Design review of the part built by this model. Coordinates are the model's own, in mm. A direction names the side the tool comes from. Coordinates: 2 decimals unless noted, no trailing zeros. Write each loop counter-clockwise with the first axis right and the second up, starting at its lowest first coordinate (ties: lowest second). Pieces come first, ordered by that corner, then holes.
Q1. Take a section at A-A (x = 29.5). Give the boundary of the cut face in (y, z), and give its area (3 significant figures).
Q2. Mouldability with a two-part tool opening along Z and no side actions: class faces 1 (the flat face through (-0.2, 17.4, 0)), 2 (the cylindrical face through (27.75, 0.99, 10.08)), 3 (the flat face through (-34, 1, 10)) as pulls with the +Z half, pulls with the -Z half, needs draft (parallel to the pull), parting line crosses it, or undercut.
Q3. Insertion check: pin 1 (3 mm diameter, centred on x = 12.5, z = 14, fed in from -Y); pin 2 (1 mm diameter, centred on y = 13, z = 4, fed in from +X); pin 3 (6 mm diameter, centred on y = 14, z = 8, fed in from -X). Each pin has a flat end and moves straight along its axis. Give the tip position at first contact, or say it passes through.
Q4. For probe 1 along Z at (x, y) = (17, 18.6); probe 2 along X at (y, z) = (14, 10); probe 3 along Z at (x, y) = (29.5, 1.5), list the stretches that pass through material, from the lowest coordinate up.
Q5. Take a section at C-C (z = 15.5). Give the boundary of the cut face in (x, y).
Q6. Take a section at B-B (z = 11). Give the boundary of the cut face in (x, y).
Q7. Take a section at D-D (x = 17). Give the boundary of the cut face in (y, z).
Q8. Machinability: for faces 4 (the flat face through (25, 11, 10)), 5 (the flat face through (-22, 9, 10)), 6 (the flat face through (-14, 19, 10)), 7 (the flat face through (-32, 2, 10)), 8 (the flat face through (34, 1, 10)), which of the approach directions +Z, -Z, +X, -X, +Y, -Y give a long, thin tool a straight path to every point of the face, cutting with its end or side? Answer none if there is none.
```python
from build123d import *

# Parameters (mm, degrees)
BOSS_EXTRUDE1_DEPTH = 20
SKETCH2_W           = 19
SKETCH2_H           = 15
CUT_EXTRUDE1_DEPTH  = 1
SKETCH3_R           = 2.5
CUT_EXTRUDE2_DEPTH  = 38.749172176
SKETCH4_W           = 9
SKETCH4_H           = 20
BOSS_EXTRUDE2_DEPTH = 2
SKETCH5_R           = 1.75
CUT_EXTRUDE3_DEPTH  = 45.226688775


with BuildPart() as part:
    # Sketch1 → Boss-Extrude1 (new body)
    with BuildSketch(Plane.XY):
        Polygon((22, 0), (22, 17), (-22, 17), (-22, 0), (-25, 0), (-25, 20), (25, 20), (25, 0), align=None)
    extrude(amount=BOSS_EXTRUDE1_DEPTH)

    # Sketch2 → Cut-Extrude1 (cut)
    with BuildSketch(Plane(origin=(0, 20, 0), x_dir=(1, 0, 0), z_dir=(0, 1, 0))):
        with Locations((-13.5, -10)):
            Rectangle(SKETCH2_W, SKETCH2_H)
    extrude(amount=-CUT_EXTRUDE1_DEPTH, mode=Mode.SUBTRACT)

    # Sketch3 → Cut-Extrude2 (cut, through all)
    with BuildSketch(Plane(origin=(0, 20, 0), x_dir=(1, 0, 0), z_dir=(0, 1, 0))):
        with Locations(Location((17, -10, 0), (0, 0, 180))):
            Circle(SKETCH3_R)
    extrude(amount=-CUT_EXTRUDE2_DEPTH, mode=Mode.SUBTRACT)

    # Sketch4 → Boss-Extrude2 (add)
    with BuildSketch(Plane.XZ):
        with Locations((-29.5, 10)):
            Rectangle(SKETCH4_W, SKETCH4_H)
        with Locations((29.5, 10)):
            Rectangle(SKETCH4_W, SKETCH4_H)
    extrude(amount=-BOSS_EXTRUDE2_DEPTH)

    # Sketch5 → Cut-Extrude3 (cut, through all)
    with BuildSketch(Plane.XZ):
        with Locations((-29.5, 10)):
            Circle(SKETCH5_R)
        with Locations((29.5, 10)):
            Circle(SKETCH5_R)
    extrude(amount=-CUT_EXTRUDE3_DEPTH, mode=Mode.SUBTRACT)


solid = part.part
```
Response:
1. outline: (0, 0) - (2, 0) - (2, 8.25) - (0, 8.25) - close; (0, 11.75) - (2, 11.75) - (2, 20) - (0, 20) - close
1. area: 33.0 mm2
2. face 1: pulls with the -Z half
2. face 2: undercut
2. face 3: needs draft
3. pin 1: stops at y = 17
3. pin 2: stops at x = 25
3. pin 3: stops at x = -25
4. probe 1: z = 0 to 7.5, 12.5 to 20
4. probe 2: x = -25 to -22, 22 to 25
4. probe 3: z = 0 to 8.25, 11.75 to 20
5. outline: (-34, 0) - (-22, 0) - (-22, 17) - (22, 17) - (22, 0) - (34, 0) - (34, 2) - (25, 2) - (25, 20) - (-4, 20) - (-4, 19) - (-23, 19) - (-23, 20) - (-25, 20) - (-25, 2) - (-34, 2) - close
6. outline: (-34, 0) - (-30.94, 0) - (-30.94, 2) - (-34, 2) - close; (-28.06, 0) - (-22, 0) - (-22, 17) - (14.71, 17) - (14.71, 20) - (-4, 20) - (-4, 19) - (-23, 19) - (-23, 20) - (-25, 20) - (-25, 2) - (-28.06, 2) - close; (19.29, 17) - (22, 17) - (22, 0) - (28.06, 0) - (28.06, 2) - (25, 2) - (25, 20) - (19.29, 20) - close; (30.94, 0) - (34, 0) - (34, 2) - (30.94, 2) - close
7. outline: (17, 0) - (20, 0) - (20, 7.5) - (17, 7.5) - close; (17, 12.5) - (20, 12.5) - (20, 20) - (17, 20) - close
8. face 4: +Z, -Z, +X, +Y
8. face 5: +Z, -Z, -Y
8. face 6: +Y
8. face 7: +Z, -Z, -X, +Y
8. face 8: +Z, -Z, +X, +Y, -Y
